Work out the finished part from the listing and answer in its coordinate system (mm). Face numbers are marked on the shaded views. Round coordinates to 2 decimals unless told otherwise and drop trailing zeros. Order: outer loops, then holes, each group sorted by start corner. A loop starts at its lowest first (then second) coordinate and runs counter-clockwise, first axis right, second up. Notation, with made-up numbers: (45.5, -38.75) - (54.5, -38.75) arc R9 cw to (54.5, -23.75) - close; hole circle Ø1 at (20, -15.75). An arc over 180 degrees is marked (long way). One line per question, with ' | ' between items. Start each with the question number.
Autodesk Inventor part; units mm, degrees
ref_plane "YZ Plane" through (0, 0, 0) normal (1, 0, 0) x (0, 1, 0)
ref_plane "XZ Plane" through (0, 0, 0) normal (0, 1, 0) x (-1, 0, 0)
ref_plane "XY Plane" through (0, 0, 0) normal (0, 0, 1) x (1, 0, 0)
sketch "Sketch1" plane through (0, 0, 0) normal (0, 0, 1) x (1, 0, 0)
  line L0 (-2, 0) -> (-4, 0)
  line L1 (-4, 92) -> (-2, 92)
  line L2 (0, 90) -> (0, 2)
  circle A0 centre (-3, 4) radius 2.075
  circle A1 centre (-3, 88) radius 2.075
  arc A2 (-4, 92) -> (-6, 90) centre (-4, 90) ccw
  arc A3 (0, 90) -> (-2, 92) centre (-2, 90) ccw
  arc A4 (-2, 0) -> (0, 2) centre (-2, 2) ccw
  arc A5 (-6, 2) -> (-4, 0) centre (-4, 2) ccw
  arc A6 (-7.5, 51.8095) -> (-7.5, 40.1905) centre (-6, 46) ccw
  circle A7 centre (-6, 46) radius 2.5
  line L3 (-6, 53.746) -> (-6, 90)
  line L4 (-6, 2) -> (-6, 38.254)
  arc A8 (-7.5, 51.8095) -> (-6, 53.746) centre (-8, 53.746) ccw
  arc A9 (-6, 38.254) -> (-7.5, 40.1905) centre (-8, 38.254) ccw
  point P0 (0, 0)
  point P1 (-6, 92)
  point P2 (-6, 0)
  point P3 (0, 92)
  point P4 (-3, 92)
  point P5 (-6, 52)
  point P6 (-6, 40)
  dimension "d0" = 6
  dimension "d1" = 92
  dimension "d2" = 4.15
  dimension "d3" = 4.15
  dimension "d4" = 84
  dimension "d5" = 4
  dimension "d6" = 2
  dimension "d12" = 12
  dimension "d13" = 5
  dimension "d14" = 2
extrude "Extrusion1" add sketch "Sketch1" along normal blind 4
chamfer "Chamfer1" distance 0.25 angle 45 28 edges at (-5.075, 88, 4) (-5.075, 88, 0) (-3, 92, 0) (-5.4142, 91.4142, 0) (-6, 71.873, 0) (-6.4189, 52.5212, 0) (-12, 46, 0) (-6.4189, 39.4788, 0) (-6, 20.127, 0) (-5.4142, 0.5858, 0) (-3, 0, 0) (-0.5858, 0.5858, 0) (0, 46, 0) (-0.5858, 91.4142, 0) (-3, 92, 4) (-5.4142, 91.4142, 4) (-6, 71.873, 4) (-6.4189, 52.5212, 4) (-12, 46, 4) (-6.4189, 39.4788, 4) (-6, 20.127, 4) (-5.4142, 0.5858, 4) (-3, 0, 4) (-0.5858, 0.5858, 4) (0, 46, 4) (-0.5858, 91.4142, 4) (-5.075, 4, 4) (-5.075, 4, 0)
equation "\"d3\" = d2"
properties part number "Spacer"
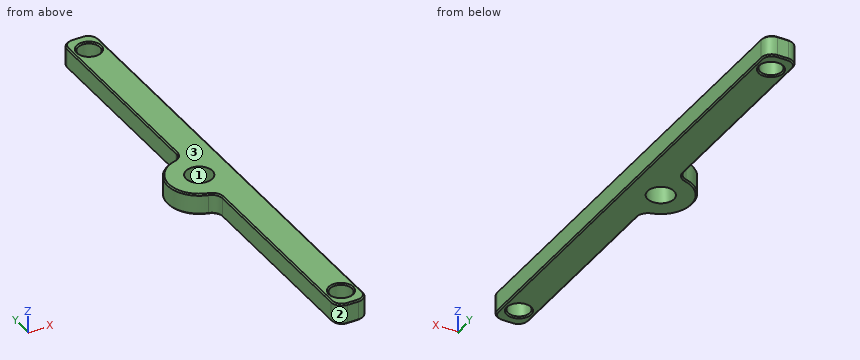
1) Section A-A on y = 46 is taken. Give the vertices of the cut face in (x, z), and give its area (3 significant figures).
2) Determine the mould class of the marked faces 1, 2 and 3 for opening direction Y: released by +Y, released by -Y, zero draft, split by the parting line, or undercut.
3) Section C-C on y = 4 is taken. Give the vertices of the cut face in (x, z) (3 decimals), and give its area (3 significant figures).
4) Section B-B on z = 0.95 is taken. Give the number of separate pieces and of enclosed holes in the cut face, and give its area (3 significant figures).
5) Straight lines are drawn through the part: line 1 (Y direction, x = -3.25, z = 1.4); line 2 (Y direction, x = -2.25, z = 0.4); line 3 (X direction, y = 69.5, z = 1.65). For each, find the intervals that lie inside material, in ascending order.
6) Section D-D on y = 20 is taken. Give the vertices of the cut face in (x, z).
7) Flat-ended cylindrical pins translate along their axes: pin 1 (1.5 mm diameter, centred on x = -10, z = 3.5, fed in from +Y); pin 2 (3 mm diameter, centred on x = -6, y = 46, fed in from +Z). Find the tip coordinate at first contact, or state that the pin passes through.
Recorded:
1) outline: (-12, 0.25) - (-11.75, 0) - (-8.5, 0) - (-8.5, 4) - (-11.75, 4) - (-12, 3.75) - close; (-3.5, 0) - (-0.25, 0) - (0, 0.25) - (0, 3.75) - (-0.25, 4) - (-3.5, 4) - close | area: 27.9 mm²
2) face 1: undercut | face 2: released by -Y | face 3: zero draft
3) outline: (-6, 0.25) - (-5.75, 0) - (-5.325, 0) - (-5.075, 0.25) - (-5.075, 3.75) - (-5.325, 4) - (-5.75, 4) - (-6, 3.75) - close; (-0.925, 0.25) - (-0.675, 0) - (-0.25, 0) - (0, 0.25) - (0, 3.75) - (-0.25, 4) - (-0.675, 4) - (-0.925, 3.75) - close | area: 7.15 mm²
4) separate pieces: 1 | enclosed holes: 3 | area: 560 mm²
5) line 1: y = 0 to 1.94, 6.06 to 85.94, 90.06 to 92 | line 2: y = 0 to 2.07, 5.93 to 86.07, 89.93 to 92 | line 3: x = -6 to 0
6) outline: (-6, 0.25) - (-5.75, 0) - (-0.25, 0) - (0, 0.25) - (0, 3.75) - (-0.25, 4) - (-5.75, 4) - (-6, 3.75) - close
7) pin 1: stops at y = 51.04 | pin 2: passes through
